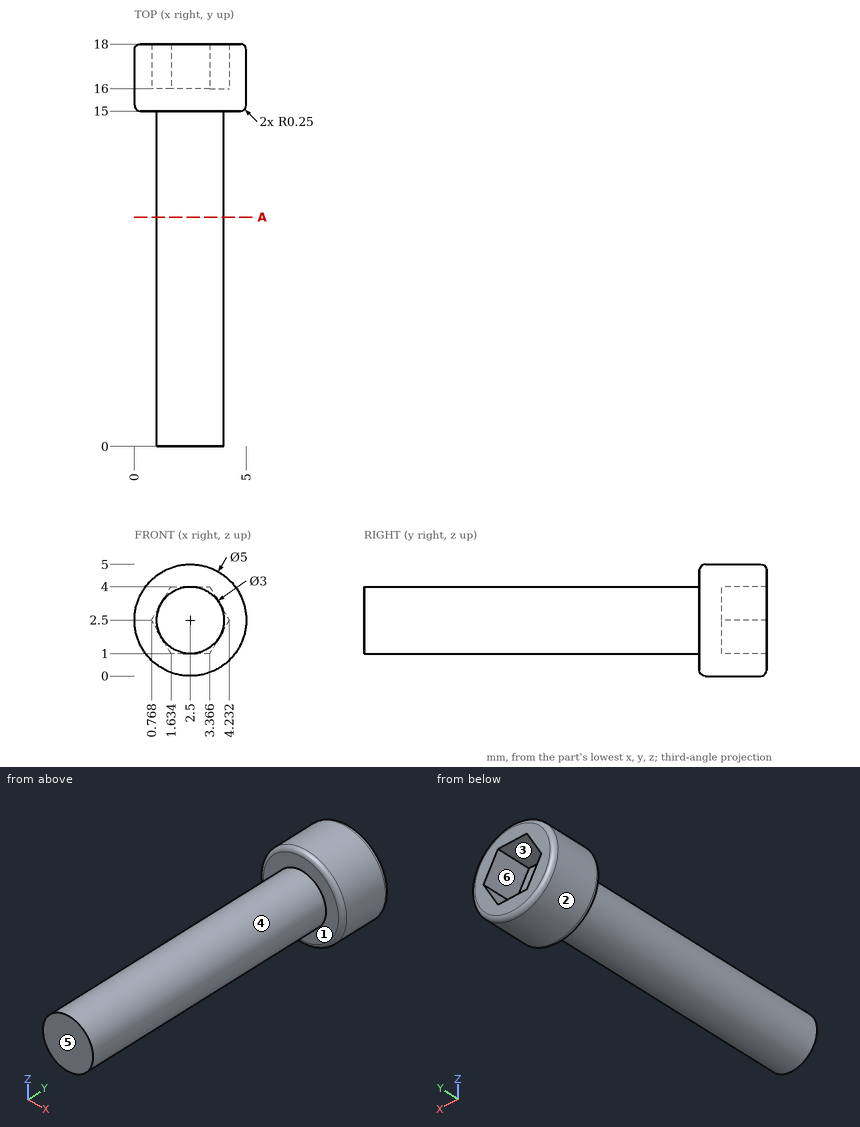
The figure shows three views and two pictorial views of one solid part (mm, origin at its lowest corner). Answer the questions. A direction names the side the tool comes from. Round coordinates to 2 decimals unless told otherwise and drop trailing zeros. Order: outer loops, then holes, each group sorted by start corner. A loop starts at its lowest first (then second) coordinate and runs counter-clockwise, first axis right, second up.
Q1. The mould has two halves that part along Z. Classify the marked faces 4, 5 and 6: pulls with the +Z half, pulls with the -Z half, needs draft (parallel to the pull), parting line crosses it, or undercut.
Solution:
face 4: parting line crosses it
face 5: needs draft
face 6: undercut
Q2. Given pin 1 Ø0.9 at (x, z) = (3, 3) entering from +Y; pin 2 Ø3 at (y, z) = (9, 3) entering from -X, each flat-ended and moving along its own axis, determine where each tip first touches the part or whether it passes through.
Solution:
pin 1: stops at y = 16
pin 2: stops at x = 1
Q3. Find the intervals of material crossed by line 1 along Y through (x, z) = (0.65, 2.3); line 2 along Y through (x, z) = (1.65, 2.15); line 3 along X through (y, z) = (8.25, 2.55), in increasing order.
Solution:
line 1: y = 15 to 18
line 2: y = 0 to 16
line 3: x = 1 to 4
Q4. A cutting plane is placed at A-A, the plane y = 10.25. Determine the outline of the cut face in (x, z).
Solution:
outline: circle Ø3 at (2.5, 2.5)
Q5. A tool of negligible diameter and unlimited length cuts with its end or side. For the marked faces 1, 2 and 3, from which of +Z, -Z, +X, -X, +Y, -Y can it reach the whole face along a straight path? Write none if from no direction.
Solution:
face 1: -Y
face 2: +Y, -Y
face 3: +Y
